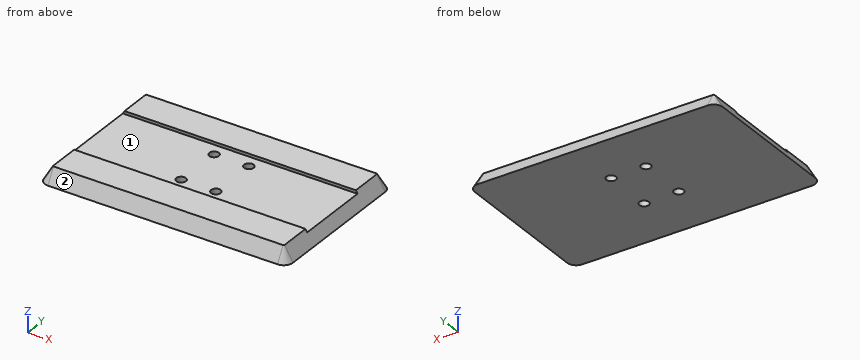
```python
from build123d import *

# Parameters (mm, degrees)
EXTRUDE_1_DEPTH        = 5
CHAMFER_2_SIZE         = 5
CHAMFER_2_SIZE_2       = 2.886751346
SKETCH_5_W             = 92.306776668
SKETCH_5_H             = 26
CUT_EXTRUDE_2_DEPTH    = 1
SKETCH_6_W             = 1
SKETCH_6_H             = 26
CUT_EXTRUDE_3_DEPTH    = 5
HOLE_WIZARD_M4_3_D     = 3.3
HOLE_WIZARD_M4_3_DEPTH = 10.1
HOLE_WIZARD_M4_3_TIP   = 0.991420021


with BuildPart() as part:
    # 草图1 → 凸台-拉伸1 (new body)
    with BuildSketch(Plane.XY):
        with BuildLine():
            Line((3.18, 0), (82.42, 0))
            ThreePointArc((82.42, 0), (84.668599564, 0.931400436), (85.6, 3.18))
            Line((85.6, 3.18), (85.6, 50.82))
            ThreePointArc((85.6, 50.82), (84.668599564, 53.068599564), (82.42, 54))
            Line((82.42, 54), (3.18, 54))
            ThreePointArc((3.18, 54), (0.931400436, 53.068599564), (0, 50.82))
            Line((0, 50.82), (0, 3.18))
            ThreePointArc((0, 3.18), (0.931400436, 0.931400436), (3.18, 0))
        make_face()
    extrude(amount=EXTRUDE_1_DEPTH)

    # 倒角2
    # the kernel refuses this chamfer: 5, 2.886751346 mm, written as the material it takes off along each edge
    with BuildSketch(Plane(origin=(85.6, 3.18, 5), x_dir=(0.019326765612699606, 0, -0.9998132206222079), z_dir=(0, 1, 0)), Plane(origin=(0, 50.82, 5), x_dir=(-0.019326765612700733, 0, -0.9998132206222079), z_dir=(0, -1, 0))) as chamfer_2_piece_1:
        Polygon((CHAMFER_2_SIZE * 0.999813220622, CHAMFER_2_SIZE * 0.0193267656127), (-CHAMFER_2_SIZE_2 * 0.0193267656124, CHAMFER_2_SIZE_2 * 0.999813220604), (0, 0), align=None)
    extrude(amount=47.64, mode=Mode.SUBTRACT)
    with BuildSketch(Plane(origin=(82.42, 50.82, 5), x_dir=(1, 0, 0), z_dir=(0, -1, 0))) as chamfer_2_piece_2:
        Polygon((3.18, -CHAMFER_2_SIZE), (3.18 - CHAMFER_2_SIZE_2, 0), (3.18, 0), align=None)
    revolve(axis=Axis((82.42, 50.82, 5), (0, 0, 1)), revolution_arc=90, mode=Mode.SUBTRACT)
    with BuildSketch(Plane(origin=(82.42, 3.18, 5), x_dir=(0, -1, 0), z_dir=(-1, 0, 0))) as chamfer_2_piece_3:
        Polygon((3.18, -CHAMFER_2_SIZE), (3.18 - CHAMFER_2_SIZE_2, 0), (3.18, 0), align=None)
    revolve(axis=Axis((82.42, 3.18, 5), (0, 0, 1)), revolution_arc=90, mode=Mode.SUBTRACT)
    with BuildSketch(Plane(origin=(82.42, 54, 5), x_dir=(0, 0.01932676561270098, -0.9998132206222079), z_dir=(-1, 0, 0)), Plane(origin=(3.18, 0, 5), x_dir=(0, -0.019326765612700754, -0.9998132206222079), z_dir=(1, 0, 0))) as chamfer_2_piece_4:
        Polygon((CHAMFER_2_SIZE * 0.999813220622, CHAMFER_2_SIZE * 0.0193267656127), (-CHAMFER_2_SIZE_2 * 0.0193267656124, CHAMFER_2_SIZE_2 * 0.999813220604), (0, 0), align=None)
    extrude(amount=79.24, mode=Mode.SUBTRACT)
    with BuildSketch(Plane(origin=(3.18, 50.82, 5), x_dir=(0, 1, 0), z_dir=(1, 0, 0))) as chamfer_2_piece_5:
        Polygon((3.18, -CHAMFER_2_SIZE), (3.18 - CHAMFER_2_SIZE_2, 0), (3.18, 0), align=None)
    revolve(axis=Axis((3.18, 50.82, 5), (0, 0, 1)), revolution_arc=90, mode=Mode.SUBTRACT)
    with BuildSketch(Plane(origin=(3.18, 3.18, 5), x_dir=(-1, 0, 0), z_dir=(0, 1, 0))) as chamfer_2_piece_6:
        Polygon((3.18, -CHAMFER_2_SIZE), (3.18 - CHAMFER_2_SIZE_2, 0), (3.18, 0), align=None)
    revolve(axis=Axis((3.18, 3.18, 5), (0, 0, 1)), revolution_arc=90, mode=Mode.SUBTRACT)

    # 草图5 → 切除-拉伸2 (cut)
    with BuildSketch(Plane.XY.offset(5)):
        with Locations((49.04013968, 27)):
            Rectangle(SKETCH_5_W, SKETCH_5_H)
    extrude(amount=-CUT_EXTRUDE_2_DEPTH, mode=Mode.SUBTRACT)

    # 草图6 → 切除-拉伸3 (cut)
    with BuildSketch(Plane(origin=(2.886751346, 0, 0), x_dir=(0, 0, -1), z_dir=(1, 0, 0))):
        with Locations((-4.5, 27)):
            Rectangle(SKETCH_6_W, SKETCH_6_H)
    extrude(amount=-CUT_EXTRUDE_3_DEPTH, mode=Mode.SUBTRACT)

    # M4 螺纹孔3
    with Locations(Plane.XY.offset(4)):
        with Locations((48.8, 18.5), (48.8, 35.5), (36.8, 18.5), (36.8, 35.5)):
            Hole(HOLE_WIZARD_M4_3_D / 2, depth=HOLE_WIZARD_M4_3_DEPTH)
            with Locations((0, 0, -(HOLE_WIZARD_M4_3_DEPTH + HOLE_WIZARD_M4_3_TIP / 2))):  # 118° drill point
                Cone(0, HOLE_WIZARD_M4_3_D / 2, HOLE_WIZARD_M4_3_TIP, mode=Mode.SUBTRACT)


solid = part.part
```
Part model, mm, in its own coordinate system. Face numbers are marked on the shaded views. A direction names the side the tool comes from. Coordinates: 2 decimals unless noted, no trailing zeros. Order: outer loops, then holes, each group sorted by start corner. A loop starts at its lowest first (then second) coordinate and runs counter-clockwise, first axis right, second up. Notation, with made-up numbers: (-28.5, 76) - (15.5, 76) arc R17 cw to (15.5, 100) - close; hole circle Ø11 at (87, -1). An arc over 180 degrees is marked (long way). Return JSON: item names as keys, results as strings. Group by question number.
Item 1: Pin check, flat tips, straight feed: pin 1 (1.5 mm diameter, centred on y = 43, z = 3.5, fed in from -X); pin 2 (0.5 mm diameter, centred on x = 28, z = 4.5, fed in from +Y); pin 3 (1.5 mm diameter, centred on x = 19, z = 3.5, fed in from +Y). Stop position of each tip, or through.
Item 2: Which spindle directions (+Z, -Z, +X, -X, +Y, -Y) get a long thin tool onto all of the face, cutting with end or side? Do the marked faces 1 and 2. Say none if no direction does.
Item 3: Cut at B-B (y = 18.5). List the corners of the cut face in (x, z).
Item 4: Cut at C-C (z = 2). List the corners of the cut face in (x, y).
Item 5: Drill centre lines: probe 1 along X at (y, z) = (36, 1.35); probe 2 along X at (y, z) = (36.5, 2.35); probe 3 along Z at (x, y) = (56, 35.5). Where is each one in solid material? Low to high. Write a range as from..to.
Item 6: Cut at D-D (y = 41). List the corners of the cut face in (x, z).
Item 7: Cut at A-A (x = 48.8). List the corners of the cut face in (y, z), plus the area to 3 significant figures.
Check values:
{
 "1": {"pin 1": "stops at x = 1.59", "pin 2": "stops at y = 51.55", "pin 3": "stops at y = 52.41"},
 "2": {"face 1": "+Z, +X, -X", "face 2": "+Z, +X, -X, -Y"},
 "3": {"outline": "(0, 0) - (35.15, 0) - (35.15, 4) - (2.31, 4) - close; (38.45, 0) - (47.15, 0) - (47.15, 4) - (38.45, 4) - close; (50.45, 0) - (85.6, 0) - (83.29, 4) - (50.45, 4) - close"},
 "4": {"outline": "(1.15, 3.18) arc R2.03 ccw to (3.18, 1.15) - (82.42, 1.15) arc R2.03 ccw to (84.45, 3.18) - (84.45, 50.82) arc R2.03 ccw to (82.42, 52.85) - (3.18, 52.85) arc R2.03 ccw to (1.15, 50.82) - close; hole circle Ø3.3 at (36.8, 18.5); hole circle Ø3.3 at (36.8, 35.5); hole circle Ø3.3 at (48.8, 18.5); hole circle Ø3.3 at (48.8, 35.5)"},
 "5": {"probe 1": "x = 0.78..35.23, 38.37..47.23, 50.37..84.82", "probe 2": "x = 1.36..35.49, 38.11..47.49, 50.11..84.24", "probe 3": "z = 0..4"},
 "6": {"outline": "(0, 0) - (85.6, 0) - (82.71, 5) - (2.89, 5) - close"},
 "7": {"outline": "(0, 0) - (16.85, 0) - (16.85, 4) - (14, 4) - (14, 5) - (2.89, 5) - close; (20.15, 0) - (33.85, 0) - (33.85, 4) - (20.15, 4) - close; (37.15, 0) - (54, 0) - (51.11, 5) - (40, 5) - (40, 4) - (37.15, 4) - close", "area": "203 mm2"}
}
